Model file for the job. Use its own axes, mm. A direction names the side the tool comes from. Coordinates: 2 decimals unless noted, no trailing zeros. Loops run counter-clockwise (first coordinate to the right, second up) from the corner with the lowest first, then second, coordinate; pieces in that order, holes last. Notation, with made-up numbers: M 59.25,41.5 L 110.25,41.5 A22 ccw 110.25,76.5 Z; hole C 44,55.25 d1. An arc over 180 degrees is marked long. One line per question, with ' | ' between items. Start each with the question number.
```python
from build123d import *

# Parameters (mm, degrees)
SKETCH1_W               = 75
SKETCH1_H               = 12.7
BOSS_EXTRUDE1_DEPTH     = 6.35
SKETCH2_R               = 5.625
CUT_EXTRUDE1_DEPTH      = 7.35
CUT_EXTRUDE1_DEPTH_BACK = 7.35
SKETCH3_W               = 23.827822186
SKETCH3_H               = 5
CUT_EXTRUDE2_DEPTH      = 7.35
CUT_EXTRUDE2_DEPTH_BACK = 7.35
M4X0_7_TAPPED_HOLE1_D   = 3.3
GOO_DEPTH               = 0.5
BOSS_EXTRUDE5_DEPTH     = 1
F_3_0MM_DOWEL_HOLE1_D   = 3
M5X0_8_TAPPED_HOLE1_D   = 4.2


with BuildPart() as part:
    # Sketch1 → Boss-Extrude1 (new body, symmetric)
    with BuildSketch(Plane(origin=(0, 0, 0), x_dir=(0, 0, -1), z_dir=(1, 0, 0))):
        Rectangle(SKETCH1_W, SKETCH1_H)
    extrude(amount=BOSS_EXTRUDE1_DEPTH, both=True)

    # Sketch2 → Cut-Extrude1 (cut, two sides)
    with BuildSketch(Plane(origin=(0, 0, 0), x_dir=(0, 0, -1), z_dir=(1, 0, 0))) as cut_extrude1_sk:
        with Locations((-6.875, 0)):
            Circle(SKETCH2_R)
        with Locations((6.875, 0)):
            Circle(SKETCH2_R)
    extrude(amount=CUT_EXTRUDE1_DEPTH, mode=Mode.SUBTRACT)
    extrude(cut_extrude1_sk.sketch, amount=-CUT_EXTRUDE1_DEPTH_BACK, mode=Mode.SUBTRACT)

    # Sketch3 → Cut-Extrude2 (cut, two sides)
    with BuildSketch(Plane(origin=(0, 0, 0), x_dir=(0, 0, -1), z_dir=(1, 0, 0))) as cut_extrude2_sk:
        Rectangle(SKETCH3_W, SKETCH3_H)
    extrude(amount=CUT_EXTRUDE2_DEPTH, mode=Mode.SUBTRACT)
    extrude(cut_extrude2_sk.sketch, amount=-CUT_EXTRUDE2_DEPTH_BACK, mode=Mode.SUBTRACT)

    # M4x0.7 Tapped Hole1 (through all)
    with Locations(Plane(origin=(0, 6.35, 0), x_dir=(1, 0, 0), z_dir=(0, 1, 0))):
        with Locations((0, 32), (0, 22), (0, -22), (0, -32)):
            Hole(M4X0_7_TAPPED_HOLE1_D / 2)

    # Sketch8 → Goo (add, symmetric)
    with BuildSketch(Plane(origin=(0, 6.35, 0), x_dir=(1, 0, 0), z_dir=(0, 1, 0))):
        with BuildLine():
            Line((-5.13731221, -8.377770681), (-5.13731221, 8.377770681))
            ThreePointArc((-5.13731221, 8.377770681), (0, 13.515082891), (5.13731221, 8.377770681))
            Line((5.13731221, 8.377770681), (5.13731221, -8.377770681))
            ThreePointArc((5.13731221, -8.377770681), (0, -13.515082891), (-5.13731221, -8.377770681))
        make_face()
    goo = extrude(amount=GOO_DEPTH, both=True)

    # Mirror1: Goo across plane
    add(goo.mirror(Plane.ZX))

    # Sketch9 → Boss-Extrude5 (add, symmetric)
    with BuildSketch(Plane(origin=(6.35, 0, 0), x_dir=(0, 0, -1), z_dir=(1, 0, 0))):
        with BuildLine():
            Line((9.451941016, -5), (27.451941016, -5))
            Line((27.451941016, -5), (27.451941016, 5))
            Line((27.451941016, 5), (9.451941016, 5))
            ThreePointArc((9.451941016, 5), (12.5, 0), (9.451941016, -5))
        make_face()
    extrude(amount=BOSS_EXTRUDE5_DEPTH, both=True)

    # Ø3.0mm Dowel Hole1 (through all)
    with Locations(Plane.ZY.offset(6.35)):
        with Locations((-22, 0), (-32, 0)):
            Hole(F_3_0MM_DOWEL_HOLE1_D / 2)

    # M5x0.8 Tapped Hole1 (through all)
    with Locations(Plane(origin=(0, 6.35, 0), x_dir=(1, 0, 0), z_dir=(0, 1, 0))):
        with Locations((0, 32), (0, 22)):
            Hole(M5X0_8_TAPPED_HOLE1_D / 2)


solid = part.part
```
(1) Band-saw the part on B-B on x = 0.5. Give the number of separate pieces and of enclosed holes in the cut face, then the cut area to 3 significant figures.
(2) Two-plate mould, pull along X, no slides. Class faces 4 (the face through (-0.969, -0.089, -20.137)), 5 (the face through (-3.88, 0.45, -33.43)), 6 (the face through (0.113, -6.603, 13.514)): pulls with the +X half, pulls with the -X half, needs draft (parallel to the pull), parting line crosses it, or undercut.
(3) Band-saw the part on D-D on z = -32. Write the cut outline in (x, y), then the cut area to 4 significant figures.
(4) Pin check, flat tips, straight feed: P1, Ø2.5, axis at y = 0, z = -22, coming from the -X side; P2, Ø0.8, axis at x = 6.5, z = -20.5, coming from the -Y side; P3, Ø5, axis at y = -2, z = 20.5, coming from the +X side; P4, Ø5.5, axis at x = 0, z = 22, coming from the +Y side. Stop position of each tip, or through.
(5) Drill centre lines: line 1 (Z direction, x = 4.2, y = 0); line 2 (Y direction, x = 6.1, z = -22); line 3 (Y direction, x = 4, z = -1). Where is each one in solid material? Low to high. Write a range as [from, to].
(6) Band-saw the part on A-A on z = 22. Write the cut outline in (x, y).
(7) 3-axis set-ups, long thin cutter, end or side, ignore diameter. For faces 1 (the face through (0.113, 6.603, 13.514)), 2 (the face through (0, -2.5, 0)), 3 (the face through (-0.113, 6.603, -13.514)): which of +Z, -Z, +X, -X, +Y, -Y reach the whole face in a straight line?
(8) Band-saw the part on C-C on z = -22. Write the cut outline in (x, y), then the cut area to 4 significant figures.
Computed values:
1) separate pieces: 5 | enclosed holes: 1 | area: 583 mm^2
2) face 4: undercut | face 5: needs draft | face 6: parting line crosses it
3) outline: M -6.35,-6.35 L -2.1,-6.35 L -2.1,-1.5 L -6.35,-1.5 Z; M -6.35,1.5 L -2.1,1.5 L -2.1,6.35 L -6.35,6.35 Z; M 2.1,-6.35 L 6.35,-6.35 L 6.35,-1.5 L 2.1,-1.5 Z; M 2.1,1.5 L 6.35,1.5 L 6.35,6.35 L 2.1,6.35 Z | area: 82.45 mm^2
4) P1: through | P2: y = -6.35 | P3: x = 6.35 | P4: y = 6.35
5) line 1: [-37.5, -33.5], [-30.5, -23.5], [-20.5, -12.5], [12.5, 37.5] | line 2: [-6.35, -1.5], [1.5, 6.35] | line 3: [-6.85, -2.5], [2.5, 6.85]
6) outline: M -6.35,-6.35 L -1.65,-6.35 L -1.65,6.35 L -6.35,6.35 Z; M 1.65,-6.35 L 6.35,-6.35 L 6.35,6.35 L 1.65,6.35 Z
7) face 1: +Z, +Y | face 2: +X, -X | face 3: -Z, +Y
8) outline: M -6.35,-6.35 L -2.1,-6.35 L -2.1,-1.5 L -6.35,-1.5 Z; M -6.35,1.5 L -2.1,1.5 L -2.1,6.35 L -6.35,6.35 Z; M 2.1,-6.35 L 6.35,-6.35 L 6.35,-5 L 7.35,-5 L 7.35,-1.5 L 2.1,-1.5 Z; M 2.1,1.5 L 7.35,1.5 L 7.35,5 L 6.35,5 L 6.35,6.35 L 2.1,6.35 Z | area: 89.45 mm^2
